Part print with two shaded views. Sizes in mm from the minimum x, y, z corner. A direction names the side the tool comes from. Give positions to 0.01 mm unless a question says otherwise; leave off trailing zeros. Write each loop counter-clockwise with the first axis right and the second up, starting at its lowest first coordinate (ties: lowest second). Pieces come first, ordered by that corner, then holes. Notation, with made-up numbers: (-35.75, 3.25) - (9.25, 3.25) arc R35 ccw to (9.25, 35.25) - close; hole circle Ø4 at (19.5, 15.25). An arc over 180 degrees is marked (long way). Answer as a JSON object with one key per item and string values.
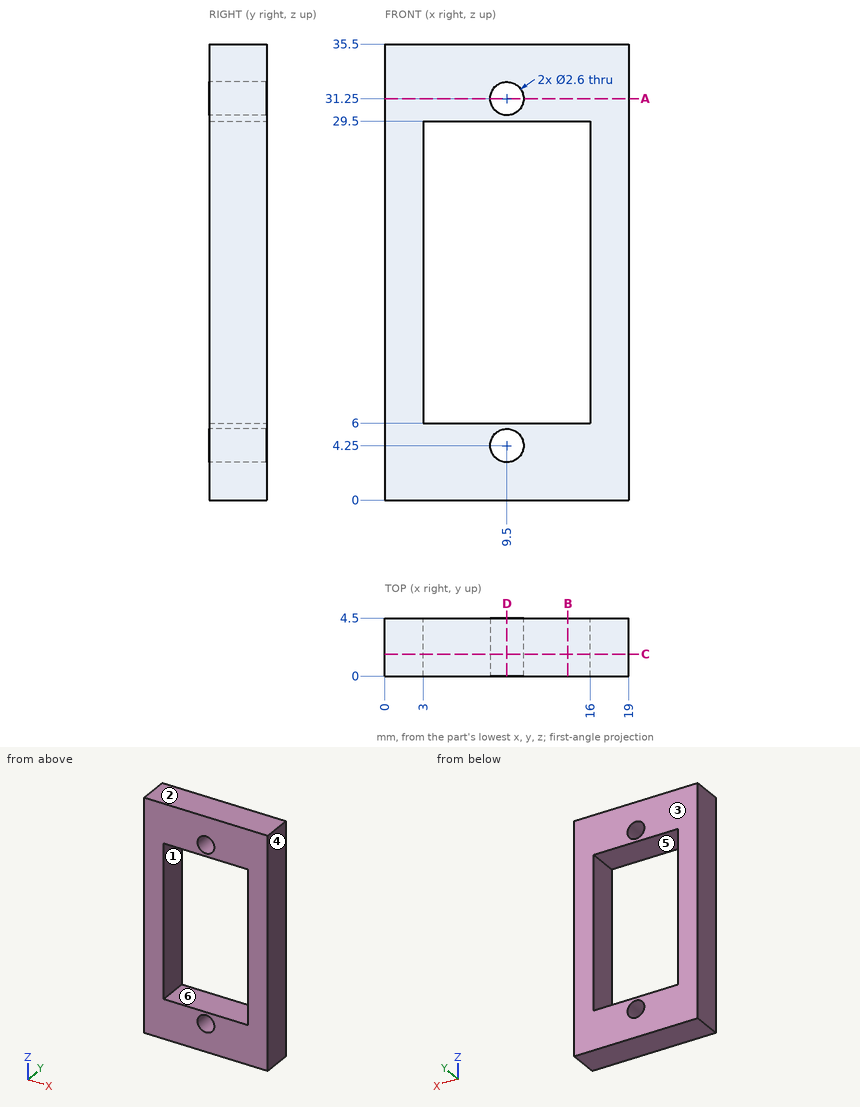
(1) Saw through at A-A, the plane z = 31.25. Give the cut face in (x, y), and give its area (3 significant figures).
Answer key:
{"outline": "(0, 0) - (8.2, 0) - (8.2, 4.5) - (0, 4.5) - close; (10.8, 0) - (19, 0) - (19, 4.5) - (10.8, 4.5) - close", "area": "73.8 mm²"}
(2) Saw through at C-C, the plane y = 1.7. Give the cut face in (x, z), and give its area (3 significant figures).
Answer key:
{"outline": "(0, 0) - (19, 0) - (19, 35.5) - (0, 35.5) - close; hole (3, 6) - (16, 6) - (16, 29.5) - (3, 29.5) - close; hole circle Ø2.6 at (9.5, 4.25); hole circle Ø2.6 at (9.5, 31.25)", "area": "358 mm²"}
(3) Saw through at D-D, the plane x = 9.5. Give the cut face in (y, z), and give its area (3 significant figures).
Answer key:
{"outline": "(0, 0) - (4.5, 0) - (4.5, 2.95) - (0, 2.95) - close; (0, 5.55) - (4.5, 5.55) - (4.5, 6) - (0, 6) - close; (0, 29.5) - (4.5, 29.5) - (4.5, 29.95) - (0, 29.95) - close; (0, 32.55) - (4.5, 32.55) - (4.5, 35.5) - (0, 35.5) - close", "area": "30.6 mm²"}
(4) Pull direction X, two halves, no side cores. Call the marked faces 3, 4, 5 and 6: pulls with the +X half, pulls with the -X half, needs draft (parallel to the pull), parting line crosses it, or undercut.
Answer key:
{"face 3": "needs draft", "face 4": "pulls with the +X half", "face 5": "undercut", "face 6": "undercut"}
(5) 3-axis set-ups, long thin cutter, end or side, ignore diameter. For the marked faces 1 and 2: which of +Z, -Z, +X, -X, +Y, -Y reach the whole face in a straight line?
Answer key:
{"face 1": "+Y, -Y", "face 2": "+Z, +X, -X, +Y, -Y"}
(6) Saw through at B-B, the plane x = 14.25. Give the cut face in (y, z), and give its area (3 significant figures).
Answer key:
{"outline": "(0, 0) - (4.5, 0) - (4.5, 6) - (0, 6) - close; (0, 29.5) - (4.5, 29.5) - (4.5, 35.5) - (0, 35.5) - close", "area": "54.0 mm²"}
(7) Flat gauge pins, fed straight in: P1, Ø2, axis at x = 11, y = 2, coming from the -Z side; P2, Ø2.5, axis at x = 9.5, z = 4.25, coming from the -Y side. Where does each tip first touch, or does it go through?
Answer key:
{"P1": "stops at z = 0", "P2": "passes through"}
(8) Probe L1, parallel to Z at x = 9.5, y = 2.95; L2, parallel to X at y = 1.3, z = 28; L3, parallel to X at y = 3.55, z = 4.25. List the from-to ranges inside material, lowest first. Write a range as [from, to].
Answer key:
{"L1": "z = [0, 2.95], [5.55, 6], [29.5, 29.95], [32.55, 35.5]", "L2": "x = [0, 3], [16, 19]", "L3": "x = [0, 8.2], [10.8, 19]"}
